CAD build for the part. Positions are in the model's coordinates, mm. Face numbers are marked on the shaded views. A direction names the side the tool comes from. Round coordinates to 2 decimals unless told otherwise and drop trailing zeros. Loops run counter-clockwise (first coordinate to the right, second up) from the corner with the lowest first, then second, coordinate; pieces in that order, holes last. Notation, with made-up numbers: M 81,-15 L 108,-15 A23 cw 108,22 Z; hole C 17,42.25 d8. An arc over 180 degrees is marked long. Use one line per item in the form item = value.
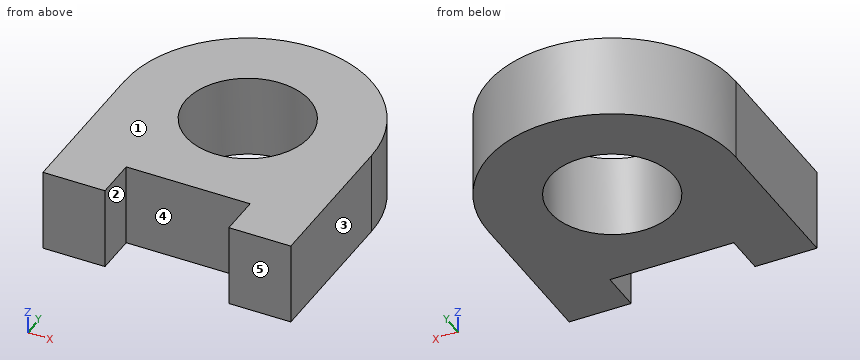
from build123d import *

# Parameters (mm, degrees)
F1_DEPTH = 508


with BuildPart() as f1:
    # F0 (on Top) → F1 (new body)
    with BuildSketch(Plane.XY):
        with BuildLine():
            Line((762, 0), (381, 0))
            ThreePointArc((381, 0), (0, -381), (-381, 0))
            Line((-381, 0), (-762, 0))
            ThreePointArc((-762, 0), (-628.132779, -431.385225), (-273.566372, -711.2))
            Line((-273.566372, -711.2), (273.566372, -711.2))
            ThreePointArc((273.566372, -711.2), (628.132779, -431.385225), (762, 0))
        make_face()
        with BuildLine():
            ThreePointArc((-273.566372, -711.2), (-628.132779, -431.385225), (-762, 0))
            Line((-762, 0), (-762, -965.2))
            Line((-762, -965.2), (-381, -965.2))
            Line((-381, -965.2), (-381, -711.2))
            Line((-381, -711.2), (-273.566372, -711.2))
        make_face()
        with BuildLine():
            Line((762, -965.2), (762, 0))
            ThreePointArc((762, 0), (628.132779, -431.385225), (273.566372, -711.2))
            Line((273.566372, -711.2), (381, -711.2))
            Line((381, -711.2), (381, -965.2))
            Line((381, -965.2), (762, -965.2))
        make_face()
        with BuildLine():
            ThreePointArc((-381, 0), (0, 381), (381, 0))
            Line((381, 0), (762, 0))
            ThreePointArc((762, 0), (0, 762), (-762, 0))
            Line((-762, 0), (-381, 0))
        make_face()
    extrude(amount=F1_DEPTH)


solid = f1.part
1. Cut at A-A on z = 420.5. Write the cut outline in (x, y), and give its area (3 significant figures).
Completed:
outline = M -762,-965.2 L -381,-965.2 L -381,-711.2 L 381,-711.2 L 381,-965.2 L 762,-965.2 L 762,0 A762 ccw -762,0 Z; hole C 0,0 d762
area = 1,730,000 mm2
2. Drop flat-ended pins along their axis: P1, Ø6, axis at y = 107, z = 341.5, coming from the +X side; P2, Ø3, axis at y = 404, z = 111.5, coming from the +X side; P3, Ø1.5, axis at y = 158.5, z = 153, coming from the -X side. Give the stop position or say it passes through.
Completed:
P1 = 754.87
P2 = 647.02
P3 = -745.49
3. Probe line 1 along Y through (x, z) = (0, 327); line 2 along X through (y, z) = (-87.5, 84); line 3 along Y through (x, z) = (-253, 419). List the from-to ranges inside material, lowest first. Write a range as from..to.
Completed:
line_1 = -711.2..-381, 381..762
line_2 = -762..-370.82, 370.82..762
line_3 = -711.2..-284.87, 284.87..718.77
4. Cut at B-B on x = 0. Write the cut outline in (y, z).
Completed:
outline = M -711.2,0 L -381,0 L -381,508 L -711.2,508 Z; M 381,0 L 762,0 L 762,508 L 381,508 Z
5. Pull direction X, two halves, no side cores. Call the marked faces 1, 2 and 3: +X half, -X half, draft (parallel to the pull), parting line (faces both ways), or undercut.
Completed:
face_1 = draft
face_2 = undercut
face_3 = +X half
6. Cut at C-C on y = -267.5. Write the cut outline in (x, z).
Completed:
outline = M -762,0 L -271.3,0 L -271.3,508 L -762,508 Z; M 271.3,0 L 762,0 L 762,508 L 271.3,508 Z
7. Tool access for the marked faces 4 and 5: list every direction of +Z, -Z, +X, -X, +Y, -Y with a clear straight run to the whole face (end or side of a thin tool).
Completed:
face_4 = +Z, -Z, -Y
face_5 = +Z, -Z, +X, -X, -Y
8. Cut at D-D on y = 550. Write the cut outline in (x, z).
Completed:
outline = M -527.39,0 L 527.39,0 L 527.39,508 L -527.39,508 Z
